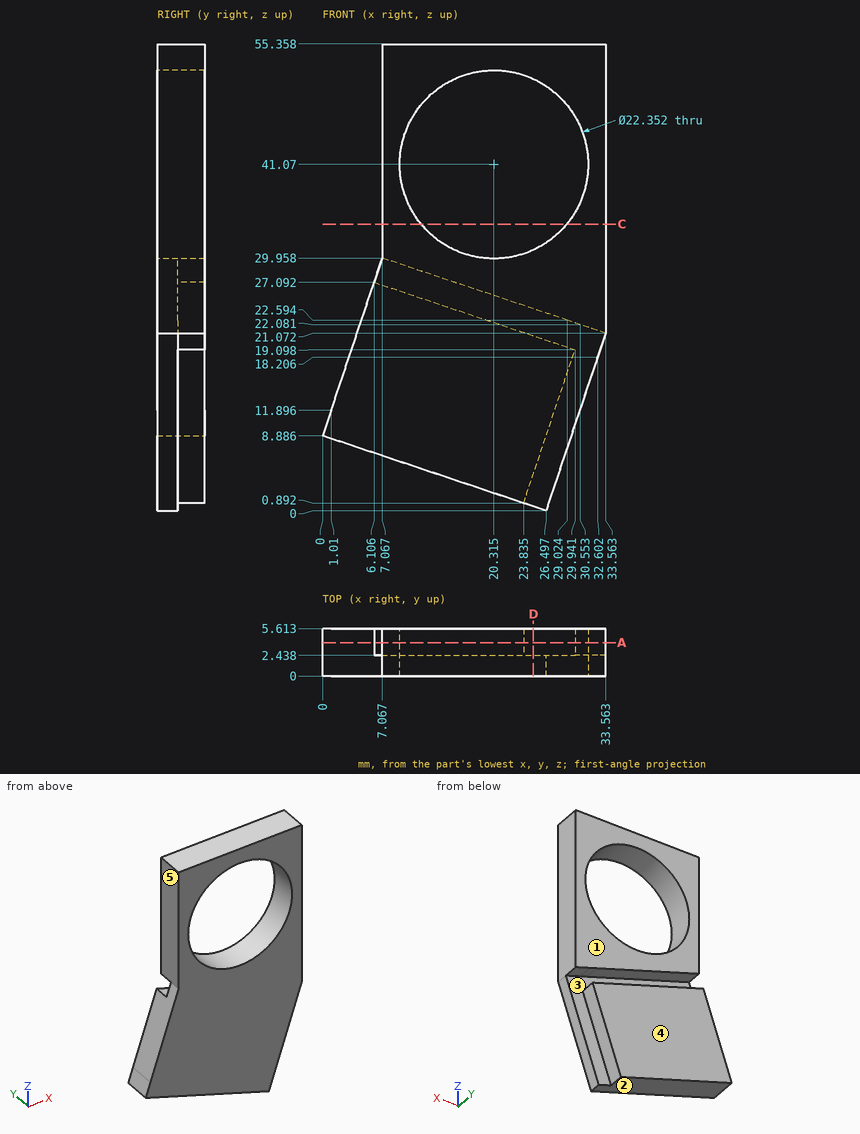
Can you work these out from the drawing? Everything is in mm from the part's minimum corner. A direction names the side the tool comes from. Round coordinates to 2 decimals unless told otherwise and drop trailing zeros. Loops run counter-clockwise (first coordinate to the right, second up) from the corner with the lowest first, then second, coordinate; pieces in that order, holes last. Notation, with made-up numbers: (56, 0.25) -> (106, 0.25) arc R17 ccw to (106, 28.25) -> close; hole circle Ø11 at (83, 58.5). An arc over 180 degrees is marked (long way). Use CSV: the item, a comma, the result in double quotes.
(1) Suppose I cut it at C-C on z = 34. Write out the boundary of the cut face in (x, y).
Return value:
outline,"(7.07, 0) -> (11.66, 0) -> (11.66, 5.61) -> (7.07, 5.61) -> close; (28.97, 0) -> (33.56, 0) -> (33.56, 5.61) -> (28.97, 5.61) -> close"
(2) Suppose I cut it at D-D on x = 25. Write out the boundary of the cut face in (y, z) (1 decimal).
Return value:
outline,"(0, 0.5) -> (2.4, 0.5) -> (2.4, 4.4) -> (5.6, 4.4) -> (5.6, 20.8) -> (2.4, 20.8) -> (2.4, 23.9) -> (5.6, 23.9) -> (5.6, 30.9) -> (0, 30.9) -> close; (0, 51.2) -> (5.6, 51.2) -> (5.6, 55.4) -> (0, 55.4) -> close"
(3) If I drill on probe 1 along Z at (x, y) = (20, 3.75); probe 2 along Z at (x, y) = (16, 4.65) (1 decimal); probe 3 along X at (y, z) = (5.2, 44), over which ranges is the centre line in solid material (lowest first)? Write a range as [from, to].
Return value:
probe 1,"z = [2.18, 22.43], [25.62, 29.9], [52.24, 55.36]"
probe 2,"z = [3.5, 23.8], [27, 30.8], [51.4, 55.4]"
probe 3,"x = [7.07, 9.53], [31.1, 33.56]"
(4) Suppose I cut it at A-A on y = 3.95. Write out the boundary of the cut face in (x, z) (1 decimal).
Return value:
outline,"(0, 8.9) -> (23.8, 0.9) -> (29.9, 19.1) -> (6.1, 27.1) -> (1, 11.9) -> close; (7.1, 30) -> (29, 22.6) -> (30.6, 22.1) -> (33.6, 21.1) -> (33.6, 55.4) -> (7.1, 55.4) -> close; hole circle Ø22.4 at (20.3, 41.1)"
(5) For the marked faces 4 and 5, which set-ups out of +Z, -Z, +X, -X, +Y, -Y let a thin tool reach every point of the face, with its end or its side?
Return value:
face 4,"+Z, -Z, +X, -X, +Y"
face 5,"+Z, -X, +Y, -Y"
(6) Will these pins go through, and if not, where does the flat tip stop? pin 1 Ø1.7 at (y, z) = (1.5, 46) entering from -X; pin 2 Ø3 at (y, z) = (2, 28) entering from -X; pin 3 Ø12 at (x, z) = (27.5, 38) entering from -Y; pin 4 Ø3 at (x, y) = (13, 4) entering from -Z.
Return value:
pin 1,"stops at x = 7.07"
pin 2,"stops at x = 5.91"
pin 3,"stops at y = 0"
pin 4,"stops at z = 4.02"
(7) If we mould it in two halves opening along X, with no side actions, what happens to the marked faces 1, 2 and 3? For each: +X half, -X half, draft (parallel to the pull), parting line (faces both ways), or undercut.
Return value:
face 1,"draft"
face 2,"-X half"
face 3,"undercut"
